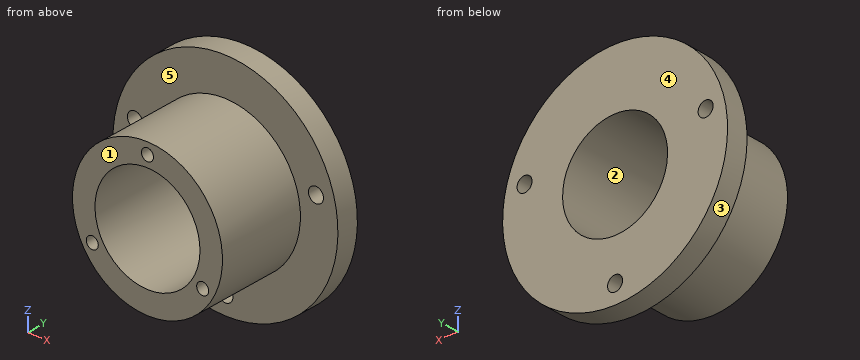
from build123d import *

# Parameters (mm, degrees)
SKETCH2_R          = 1
CUT_EXTRUDE1_DEPTH = 26.980762114
SKETCH3_R          = 0.8
CUT_EXTRUDE2_DEPTH = 2.5


with BuildPart() as part:
    # Sketch1 → Revolve1 (revolve)
    with BuildSketch(Plane.XY, mode=Mode.PRIVATE) as revolve1_sk:
        Polygon((10, 0), (10, 12), (15, 12), (15, 15), (7, 15), (7, 0), align=None)
    revolve(revolve1_sk.sketch.rotate(Axis((0, 0, 0), (0, 1, 0)), 90), axis=Axis((0, 0, 0), (0, 1, 0)))

    # Sketch2 → Cut-Extrude1 (cut, through all)
    with BuildSketch(Plane(origin=(0, 15, 0), x_dir=(1, 0, 0), z_dir=(0, 1, 0))):
        with Locations(Location((0, 12.5, 0), (0, 0, 270))):
            Circle(SKETCH2_R)
        with Locations(Location((-12.074072829, -3.235238064, 0), (0, 0, 270))):
            Circle(SKETCH2_R)
        with Locations(Location((12.074072829, -3.235238064, 0), (0, 0, 270))):
            Circle(SKETCH2_R)
    extrude(amount=-CUT_EXTRUDE1_DEPTH, mode=Mode.SUBTRACT)

    # Sketch3 → Cut-Extrude2 (cut)
    with BuildSketch(Plane.XZ):
        with Locations(Location((0, 8.5, 0), (0, 0, 270))):
            Circle(SKETCH3_R)
        with Locations(Location((7.361215932, -4.25, 0), (0, 0, 270))):
            Circle(SKETCH3_R)
        with Locations(Location((-7.361215932, -4.25, 0), (0, 0, 270))):
            Circle(SKETCH3_R)
    extrude(amount=-CUT_EXTRUDE2_DEPTH, mode=Mode.SUBTRACT)


solid = part.part
Verification items for the finished model (mm, model axes). Face numbers are marked on the shaded views. A direction names the side the tool comes from. Give positions to 0.01 mm unless a question says otherwise; leave off trailing zeros. Loops run counter-clockwise (first coordinate to the right, second up) from the corner with the lowest first, then second, coordinate; pieces in that order, holes last. Notation, with made-up numbers: (35, -14) - (84, -14) arc R13 cw to (84, 9) - close; hole circle Ø8 at (59.5, 15.5). An arc over 180 degrees is marked (long way). Write each question's results on one line, items separated by ' | '.
1) Sectioned sample at C-C on x = 5.5. Record the boundary of the cut face in (y, z), plus the area to 3 significant figures.
Solution:
outline: (0, -8.35) - (12, -8.35) - (12, -13.96) - (15, -13.96) - (15, -4.33) - (0, -4.33) - close; (0, 4.33) - (15, 4.33) - (15, 13.96) - (12, 13.96) - (12, 8.35) - (0, 8.35) - close | area: 154 mm2
2) Material ranges on L1, parallel to X at y = 6.25, z = 0; L2, parallel to Z at x = -0.5, y = 1.75; L3, parallel to X at y = 1.6, z = -4.25, recorded low to high. Write a range as from..to.
Solution:
L1: -10..-7, 7..10 | L2: -9.99..-6.98, 6.98..7.88, 9.12..9.99 | L3: -9.05..-8.16, -6.56..-5.56, 5.56..6.56, 8.16..9.05
3) Depth check by flat-ended pin: P1, Ø1.8, axis at x = 7, z = -4, coming from the -Y side; P2, Ø4, axis at y = 7.5, z = 4, coming from the -X side; P3, Ø12.5, axis at x = 0, z = 0, coming from the -Y side; P4, Ø2.5, axis at x = -12.07, z = 3.24, coming from the -Y side. Enter the tip coordinate at first touch or a pass-through.
Solution:
P1: y = 0 | P2: x = -9.8 | P3: through | P4: y = 12
4) Tool access check on the marked faces 4 and 5. Record the directions out of +Z, -Z, +X, -X, +Y, -Y that give a thin tool (end or side, any length) a straight path to the whole face; none if there is none.
Solution:
face 4: +Z, -Z, +X, -X, +Y | face 5: -Y
5) Mould release check, pull along Z, two halves, no side actions. Record for the marked faces 1, 2 and 3: pulls with the +Z half, pulls with the -Z half, needs draft (parallel to the pull), parting line crosses it, or undercut.
Solution:
face 1: needs draft | face 2: undercut | face 3: parting line crosses it
6) Sectioned sample at A-A on x = 0. Record the boundary of the cut face in (y, z).
Solution:
outline: (0, -10) - (12, -10) - (12, -11.5) - (15, -11.5) - (15, -7) - (0, -7) - close; (0, 7) - (15, 7) - (15, 15) - (12, 15) - (12, 10) - (0, 10) - (0, 9.3) - (2.5, 9.3) - (2.5, 7.7) - (0, 7.7) - close; (12, -15) - (15, -15) - (15, -13.5) - (12, -13.5) - close
7) Sectioned sample at D-D on y = 10. Record the boundary of the cut face in (x, z).
Solution:
outline: circle Ø20 at (0, 0); hole circle Ø14 at (0, 0)
8) Sectioned sample at B-B on z = 0. Record the boundary of the cut face in (x, y), plus the area to 3 significant figures.
Solution:
outline: (-15, 12) - (-10, 12) - (-10, 0) - (-7, 0) - (-7, 15) - (-15, 15) - close; (7, 0) - (10, 0) - (10, 12) - (15, 12) - (15, 15) - (7, 15) - close | area: 120 mm2
